```python
from build123d import *

# Parameters (mm, degrees)
SKETCH_W                = 23
SKETCH_H                = 23
PAD_DEPTH               = 2
PAD001_DEPTH            = 7.5
SKETCH016_R             = 1.5
POCKET_DEPTH            = 7.25
SKETCH012_R             = 1.75
POCKET001_DEPTH         = 5
PAD002_DEPTH            = 2
CHAMFER_SIZE            = 1
BODY001_PLACEMENT_ANGLE = 180


with BuildPart() as part:
    # Sketch → Pad (new body)
    with BuildSketch(Plane.YZ):
        Rectangle(SKETCH_W, SKETCH_H)
    extrude(amount=PAD_DEPTH)

    # Sketch017 (on Face4 of Pad) → Pad001 (join)
    with BuildSketch(Plane(origin=(0, 0, 11.5), x_dir=(0, -1, 0), z_dir=(0, 0, 1))):
        Polygon((-15, -23.23103), (15, -23.23103), (17, -9.88), (15, 2), (-15, 2), (-17, -9.88), align=None)
    extrude(amount=PAD001_DEPTH)

    # Sketch016 (on Face13 of Pad001) → Pocket (cut)
    with BuildSketch(Plane(origin=(0, 0, 19), x_dir=(0, -1, 0), z_dir=(0, 0, 1))):
        with Locations((11.75, -2.18)):
            Circle(SKETCH016_R)
        with Locations((-11.75, -2.18)):
            Circle(SKETCH016_R)
    extrude(amount=-POCKET_DEPTH, mode=Mode.SUBTRACT)

    # Sketch012 (on Face4 of Pad001) → Pocket001 (cut)
    with BuildSketch(Plane(origin=(0, 0, 0), x_dir=(0, 1, 0), z_dir=(-1, 0, 0))):
        with Locations((-4.75, -4.735)):
            Circle(SKETCH012_R)
        with Locations((4.75, 4.735)):
            Circle(SKETCH012_R)
    extrude(amount=-POCKET001_DEPTH, mode=Mode.SUBTRACT)

    # Sketch018 (on Face1 of Pocket001) → Pad002 (join)
    with BuildSketch(Plane(origin=(0, -11.5, 0), x_dir=(0, 0, -1), z_dir=(0, -1, 0))):
        Polygon((-11.5, -9.88), (11.5, 0), (-11.5, 0), align=None)
    pad002 = extrude(amount=-PAD002_DEPTH)

    # Mirrored: Pad002 across XZ
    add(pad002.mirror(Plane.XZ))

    # Chamfer
    chamfer_edges = [part.edges().sort_by_distance(p)[0] for p in [
        (-2.18, 13.25, 19),
        (-2.18, -10.25, 19),
    ]]
    chamfer(chamfer_edges, length=CHAMFER_SIZE)


with BuildPart() as part_1:
    # Body001 placement: moved
    add(part.part.rotate(Axis((0, 0, 0), (1, 0, 0)), BODY001_PLACEMENT_ANGLE))


solid = part_1.part
```
Geometry: final body of the model. Coordinates: model frame, mm. A direction names the side the tool comes from. Round coordinates to 2 decimals unless told otherwise and drop trailing zeros. Loops run counter-clockwise (first coordinate to the right, second up) from the corner with the lowest first, then second, coordinate; pieces in that order, holes last.
Item 1: Section A-A, the plane y = 4.75. Output: boundary loops of the cut face in (x, z) (3 decimals), plus the area to 3 significant figures.
Checked values:
outline: (-23.231, -19) - (2, -19) - (2, -6.485) - (0, -6.485) - (0, -11.5) - (-23.231, -11.5) - close; (0, -2.985) - (2, -2.985) - (2, 11.5) - (0, 11.5) - close
area: 228 mm2
Item 2: Section B-B, the plane z = -13. Output: boundary loops of the cut face in (x, y).
Checked values:
outline: (-23.23, -15) - (-9.88, -17) - (2, -15) - (2, 15) - (-9.88, 17) - (-23.23, 15) - close; hole circle Ø3 at (-2.18, -11.75); hole circle Ø3 at (-2.18, 11.75)
Item 3: Mould query, pull axis Z, two halves, no side actions, for faces 1 (the flat face through (-2, -12, -11.75)), 2 (the cylindrical face through (-2.11, 10.25, -14.92)), 3 (the cylindrical face through (0.986, 5.129, -6.443)), 4 (the cylindrical face through (1, -3, 4.8)). Classes: released by +Z, released by -Z, zero draft, split by the parting line, or undercut.
Checked values:
face 1: released by -Z
face 2: zero draft
face 3: undercut
face 4: undercut
Item 4: Contact query for flat-ended pins moving along their axis: P1, Ø3.5, axis at x = -3.5, z = -1.5, coming from the +Y side; P2, Ø5, axis at x = -4.5, z = -3.5, coming from the -Y side; P3, Ø5, axis at y = 5, z = 4, coming from the -X side; P4, Ø5, axis at y = -8.5, z = -10.5, coming from the -X side. Output: stop coordinate, or through.
Checked values:
P1: stops at y = 11.5
P2: stops at y = -11.5
P3: stops at x = 0
P4: stops at x = -23.23
Item 5: Line query: L1, parallel to Y at x = -4.75, z = -4.5; L2, parallel to Z at x = 0.45, y = -4.75 (3 decimals); L3, parallel to X at y = 11.75, z = -14.75. Output: solid intervals per line, ascending.
Checked values:
L1: y = -11.5 to -9.5, 9.5 to 11.5
L2: z = -19 to 2.985, 6.485 to 11.5
L3: x = -23.23 to -3.68, -0.68 to 2
Item 6: Section D-D, the plane x = -8.5. Output: boundary loops of the cut face in (y, z).
Checked values:
outline: (-16.77, -19) - (16.77, -19) - (16.77, -11.5) - (11.5, -11.5) - (11.5, -8.29) - (9.5, -8.29) - (9.5, -11.5) - (-9.5, -11.5) - (-9.5, -8.29) - (-11.5, -8.29) - (-11.5, -11.5) - (-16.77, -11.5) - close
Item 7: Reachability of faces 5 (the cylindrical face through (-2.11, -13.25, -14.92)), 6 (the flat face through (-10, 0, -11.5)), 7 (the flat face through (-3, 11.5, -3)), 8 (the flat face through (-16.649, 15.986, -15.198)), 9 (the flat face through (-10, 0, -19)) from +Z, -Z, +X, -X, +Y, -Y: full face, straight path, thin tool, end or side. Return the list, or none.
Checked values:
face 5: -Z
face 6: +Z, -X
face 7: +Z, +X, -X, +Y
face 8: +Z, -Z, -X, +Y
face 9: -Z, +X, -X, +Y, -Y
Item 8: Section C-C, the plane z = -4. Output: boundary loops of the cut face in (x, y), plus the area to 3 significant figures.
Checked values:
outline: (-6.66, -11.5) - (2, -11.5) - (2, 3.16) - (0, 3.16) - (0, -9.5) - (-6.66, -9.5) - close; (-6.66, 9.5) - (0, 9.5) - (0, 6.34) - (2, 6.34) - (2, 11.5) - (-6.66, 11.5) - close
area: 66.3 mm2
